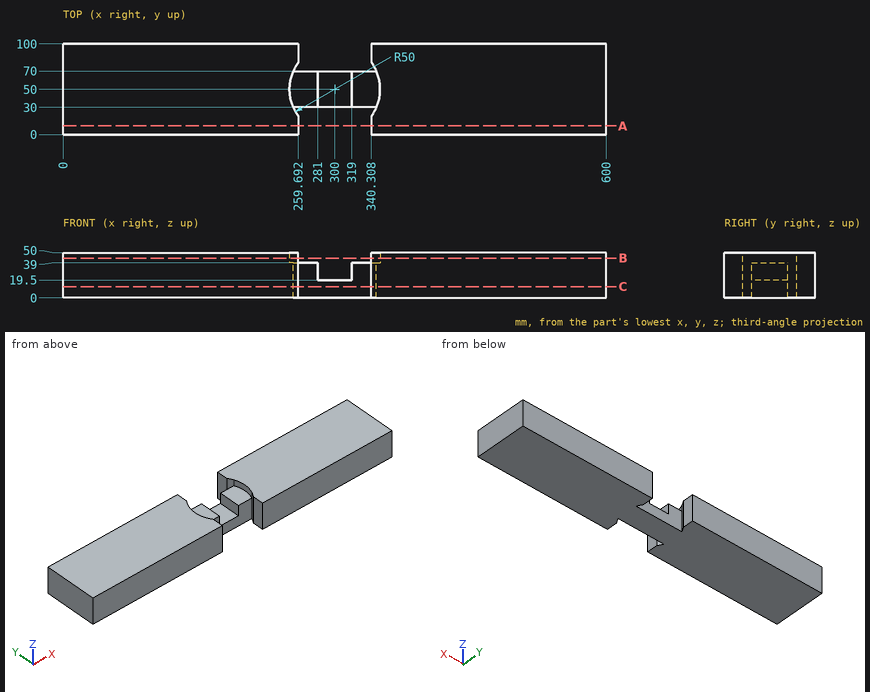
Can you work these out from the drawing? Everything is in mm from the part's minimum corner. Give positions to 0.01 mm unless a question says otherwise; leave off trailing zeros. Order: outer loops, then holes, each group sorted by start corner. A loop starts at its lowest first (then second) coordinate and runs counter-clockwise, first axis right, second up. Notation, with made-up numbers: (23.5, -5) -> (64.5, -5) arc R22 ccw to (64.5, 17) -> close; hole circle Ø11 at (-20, 36.25). An arc over 180 degrees is marked (long way). Return JSON: item names as keys, results as strings.
1. I need wall thicknesses on line 1 (X direction, y = 92.5, z = 20.5); line 2 (X direction, y = 47.5, z = 35); line 3 (Y direction, x = 300, z = 8). Which ranges of each line are inside material? Lowest first, please. Write a range as from..to.
Answer list:
{"line 1": "x = 0..259.69, 340.31..600", "line 2": "x = 0..281, 319..600", "line 3": "y = 30..70"}
2. Imagine slicing it at A-A on y = 9.5. List the corners of the cut face in (x, z) for me, then the cut area to 3 significant figures.
Answer list:
{"outline": "(0, 0) -> (259.69, 0) -> (259.69, 50) -> (0, 50) -> close; (340.31, 0) -> (600, 0) -> (600, 50) -> (340.31, 50) -> close", "area": "26,000 mm2"}
3. For pin 1 Ø19.5 at (x, z) = (310.5, 14.5) entering from +Y; pin 2 Ø15.5 at (x, y) = (332.5, 46) entering from +Z, each with a flat end and sliding along its axis, tell me the tip position at first contact or that it passes through.
Answer list:
{"pin 1": "stops at y = 70", "pin 2": "stops at z = 39"}
4. Imagine slicing it at B-B on z = 44. List the corners of the cut face in (x, y) for me (3 decimals).
Answer list:
{"outline": "(0, 0) -> (259.692, 0) -> (259.692, 20.415) arc R50 cw to (259.692, 79.585) -> (259.692, 100) -> (0, 100) -> close; (340.308, 0) -> (600, 0) -> (600, 100) -> (340.308, 100) -> (340.308, 79.585) arc R50 cw to (340.308, 20.415) -> close"}
5. Imagine slicing it at C-C on z = 12.5. List the corners of the cut face in (x, y) for me (3 decimals), then the cut area to 3 significant figures.
Answer list:
{"outline": "(0, 0) -> (259.692, 0) -> (259.692, 20.415) arc R50 cw to (254.174, 30) -> (345.826, 30) arc R50 cw to (340.308, 20.415) -> (340.308, 0) -> (600, 0) -> (600, 100) -> (340.308, 100) -> (340.308, 79.585) arc R50 cw to (345.826, 70) -> (254.174, 70) arc R50 cw to (259.692, 79.585) -> (259.692, 100) -> (0, 100) -> close", "area": "55,000 mm2"}
